Could you check a few things on this model? Use its own coordinates, in mm. Face numbers are marked on the shaded views. A direction names the side the tool comes from. Round coordinates to 2 decimals unless told otherwise and drop trailing zeros. Order: outer loops, then holes, each group sorted by start corner. A loop starts at its lowest first (then second) coordinate and runs counter-clockwise, first axis right, second up.
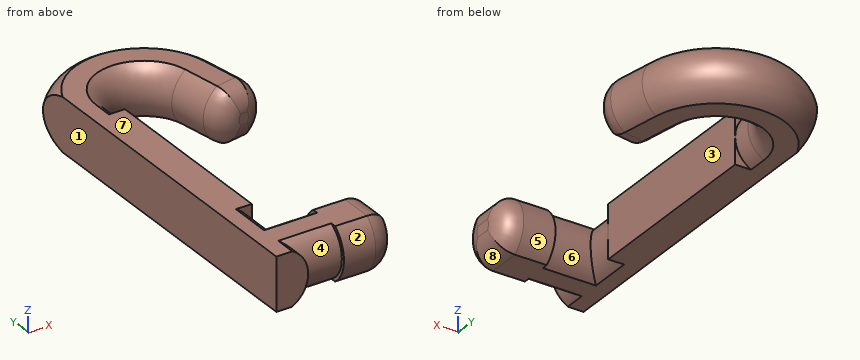
```python
from build123d import *

# Parameters (mm, degrees)
EXTRUDE_1_DEPTH     = 5
SKETCH_19_W         = 5
SKETCH_19_H         = 18
EXTRUDE_2_DEPTH     = 1.5
FILLET_2_R          = 2
SKETCH_20_W         = 8
SKETCH_20_H         = 40
CUT_EXTRUDE_1_DEPTH = 36.961786675


with BuildPart() as part:
    # 扫描2: sweep along a path in 草图1
    with BuildLine(Plane.XY) as sweep_2_path:
        Line((11.886241035, 20.255064977), (10.916442642, 25.755064977))
        ThreePointArc((10.916442642, 25.755064977), (5.020643415, 30.27907084), (0, 24.8))
        Line((0, 24.8), (0, 0))
        Line((0, 0), (0, -3))
    # 草图13 → 扫描2 (sweep)
    with BuildSketch(Plane(origin=(0, -3, 0), x_dir=(1, 0, 0), z_dir=(0, 1, 0))):
        with BuildLine():
            Line((-1, -2.5), (1, -2.5))
            ThreePointArc((1, -2.5), (2.5, 0), (1, 2.5))
            Line((1, 2.5), (-1, 2.5))
            ThreePointArc((-1, 2.5), (-2.5, 0), (-1, -2.5))
        make_face()
    sweep(path=sweep_2_path.line)

    # 扫描4: sweep along a path in 草图15
    with BuildLine(Plane.XY) as sweep_4_path:
        Line((0, 0), (11, 0))
    # 草图16 → 扫描4 (sweep)
    with BuildSketch(Plane(origin=(11, 0, 0), x_dir=(0, 0, -1), z_dir=(1, 0, 0))):
        with BuildLine():
            Line((-2.5, -1), (-2.5, 1))
            ThreePointArc((-2.5, 1), (0, 2.5), (2.5, 1))
            Line((2.5, 1), (2.5, -1))
            ThreePointArc((2.5, -1), (0, -2.5), (-2.5, -1))
        make_face()
    sweep(path=sweep_4_path.line)

    # 草图17 → 凸台-拉伸1 (add)
    with BuildSketch(Plane(origin=(11, 0, 0), x_dir=(0, 0, -1), z_dir=(1, 0, 0))):
        with BuildLine():
            Line((-2.5, 1.555522876), (-2.5, -1.555522876))
            ThreePointArc((-2.5, -1.555522876), (0, -2.8), (2.5, -1.555522876))
            Line((2.5, -1.555522876), (2.5, 1.555522876))
            ThreePointArc((2.5, 1.555522876), (0, 2.8), (-2.5, 1.555522876))
        make_face()
    extrude(amount=-EXTRUDE_1_DEPTH)

    # 草图19 → 凸台-拉伸2 (add)
    with BuildSketch(Plane(origin=(1, 0, 0), x_dir=(0, 0, -1), z_dir=(1, 0, 0))):
        with Locations((0, 14)):
            Rectangle(SKETCH_19_W, SKETCH_19_H)
    extrude(amount=EXTRUDE_2_DEPTH)

    # 圆角2
    # the kernel refuses this fillet: 2 mm, written as the material it takes off along each edge
    with BuildSketch(Plane(origin=(17.795087554, 21.296954043, 2.5), x_dir=(0, 0, -1), z_dir=(-0.9848077530122092, -0.17364817766692373, 0))) as fillet_2_piece_1:
        with BuildLine():
            CenterArc((FILLET_2_R, -FILLET_2_R), FILLET_2_R, 90, 90)
            Line((0, -FILLET_2_R), (0, 0))
            Line((0, 0), (FILLET_2_R, 0))
        make_face()
    extrude(amount=12, mode=Mode.SUBTRACT)
    with BuildSketch(Plane(origin=(12.214510286, 20.312947703, 0), x_dir=(0.9423506208781959, 0.16616183974819204, -0.29045748456869663), z_dir=(0.2860447827236766, 0.05043741288507259, 0.9568878981667733))) as fillet_2_piece_2:
        with BuildLine():
            CenterArc((2.833333333 - FILLET_2_R, FILLET_2_R), FILLET_2_R, 270, 90)
            Line((2.833333333 - FILLET_2_R, 0), (2.833333333, 0))
            Line((2.833333333, 0), (2.833333333, FILLET_2_R))
        make_face()
    revolve(axis=Axis((12.214510286, 20.312947703, 0), (-0.173648177666923, 0.9848077530122094, 0)), revolution_arc=326.229306127, mode=Mode.SUBTRACT)
    with BuildSketch(Plane(origin=(5.977394517, 19.213175911, -2.5), x_dir=(-0.17364817766692373, 0.9848077530122092, 0), z_dir=(0.9848077530122092, 0.17364817766692373, 0))) as fillet_2_piece_3:
        with BuildLine():
            CenterArc((FILLET_2_R, FILLET_2_R), FILLET_2_R, 180, 90)
            Line((0, FILLET_2_R), (0, 0))
            Line((0, 0), (FILLET_2_R, 0))
        make_face()
    extrude(amount=12, mode=Mode.SUBTRACT)
    with BuildSketch(Plane(origin=(11, -6.555522876, 2.5), x_dir=(0, 0, -1), z_dir=(0, 1, 0))) as fillet_2_piece_4:
        with BuildLine():
            CenterArc((FILLET_2_R, FILLET_2_R), FILLET_2_R, 180, 90)
            Line((0, FILLET_2_R), (0, 0))
            Line((0, 0), (FILLET_2_R, 0))
        make_face()
    extrude(amount=13.111045751, mode=Mode.SUBTRACT)
    with BuildSketch(Plane(origin=(11, 6.555522876, -2.5), x_dir=(-1, 0, 0), z_dir=(0, -1, 0))) as fillet_2_piece_5:
        with BuildLine():
            CenterArc((FILLET_2_R, -FILLET_2_R), FILLET_2_R, 90, 90)
            Line((0, -FILLET_2_R), (0, 0))
            Line((0, 0), (FILLET_2_R, 0))
        make_face()
    extrude(amount=13.111045751, mode=Mode.SUBTRACT)
    with BuildSketch(Plane(origin=(11, -0.333333333, 0), x_dir=(0, -0.8131785022115455, -0.582014367125922), z_dir=(0, -0.582014367125922, 0.8131785022115455))) as fillet_2_piece_6:
        with BuildLine():
            CenterArc((3.133333333 - FILLET_2_R, -FILLET_2_R), FILLET_2_R, 0, 90)
            Line((3.133333333, -FILLET_2_R), (3.133333333, 0))
            Line((3.133333333, 0), (3.133333333 - FILLET_2_R, 0))
        make_face()
    revolve(axis=Axis((11, -0.333333333, 0), (1, 0, 0)), revolution_arc=288.815304863, mode=Mode.SUBTRACT)
    with BuildSketch(Plane(origin=(11, 0.333333333, 0), x_dir=(0, 0.8131785022115376, 0.5820143671259329), z_dir=(0, 0.5820143671259329, -0.8131785022115376))) as fillet_2_piece_7:
        with BuildLine():
            CenterArc((3.133333333 - FILLET_2_R, -FILLET_2_R), FILLET_2_R, 0, 90)
            Line((3.133333333 - FILLET_2_R, 0), (3.133333333, 0))
            Line((3.133333333, 0), (3.133333333, -FILLET_2_R))
        make_face()
    revolve(axis=Axis((11, 0.333333333, 0), (1, 0, 0)), revolution_arc=288.815304863, mode=Mode.SUBTRACT)
    with BuildSketch(Plane(origin=(11.557971784, 20.197182251, 0), x_dir=(-0.9423506208781961, -0.16616183974819207, 0.2904574845686964), z_dir=(-0.2860447827236764, -0.05043741288507257, -0.9568878981667737))) as fillet_2_piece_8:
        with BuildLine():
            CenterArc((2.833333333 - FILLET_2_R, FILLET_2_R), FILLET_2_R, 270, 90)
            Line((2.833333333, FILLET_2_R), (2.833333333, 0))
            Line((2.833333333, 0), (2.833333333 - FILLET_2_R, 0))
        make_face()
    revolve(axis=Axis((11.557971784, 20.197182251, 0), (-0.17364817766692306, 0.9848077530122095, 0)), revolution_arc=326.229306127, mode=Mode.SUBTRACT)

    # 草图20 → 切除-拉伸1 (cut, through all)
    with BuildSketch(Plane(origin=(-0.5, 0, 0), x_dir=(0, 0, -1), z_dir=(1, 0, 0))):
        with Locations((0, 16)):
            Rectangle(SKETCH_20_W, SKETCH_20_H)
    extrude(amount=-CUT_EXTRUDE_1_DEPTH, mode=Mode.SUBTRACT)


solid = part.part
```
Q1. We'd pull the mould along Y, two halves only. Please class the marked faces 1, 2 and 3: released by +Y, released by -Y, zero draft, split by the parting line, or undercut.
Q2. For P1, Ø2, axis at y = 19, z = 0, coming from the +X side; P2, Ø0.8, axis at y = -0.5, z = 0, coming from the +X side; P3, Ø0.5, axis at x = 2, z = 1.5, coming from the +Y side, each with a flat end and sliding along its axis, tell me the tip position at first contact or that it passes through.
Q3. For the marked faces 4, 5, 6, 7 and 8, which set-ups out of +Z, -Z, +X, -X, +Y, -Y let a thin tool reach every point of the face, with its end or its side?
Q4. Imagine slicing it at A-A, the plane y = 12.5. Please give me the cut outline in (x, z), then the cut area to 3 significant figures.
Q5. I need wall thicknesses on L1, parallel to X at y = 11, z = -1.95; L2, parallel to Y at x = 8.25, z = -0.85; L3, parallel to Y at x = 7.25, z = 0.45. Which ranges of each line are inside material? Lowest first, please.
Filled in:
1. face 1: zero draft
1. face 2: released by -Y
1. face 3: undercut
2. P1: stops at x = 2.5
2. P2: stops at x = 11
2. P3: stops at y = 31.72
3. face 4: -Y
3. face 5: +X
3. face 6: none
3. face 7: +Z, +X, -X, +Y, -Y
3. face 8: -Z, +X, -Y
4. outline: (-0.5, -2.5) - (2.5, -2.5) - (2.5, 2.5) - (-0.5, 2.5) - close
4. area: 15.0 mm2
5. L1: x = -0.5 to 2.5
5. L2: y = -2.68 to 2.68, 26.3 to 32.17
5. L3: y = -2.77 to 2.77, 27.28 to 32.57
